```python
from build123d import *

# Parameters (mm, degrees)
ESQUISSE1_R                  = 100
BOSS_EXTRU_1_DEPTH           = 10
ENL_V_MAT_EXTRU_1_DEPTH      = 142.774468788
ENL_V_MAT_EXTRU_1_DEPTH_BACK = 142.774468788
CONG_1_R                     = 5
ENL_V_MAT_EXTRU_2_DEPTH      = 142.774468788
ENL_V_MAT_EXTRU_2_DEPTH_BACK = 142.774468788
ESQUISSE3_R                  = 8
ENL_V_MAT_EXTRU_3_DEPTH      = 142.774468788
ENL_V_MAT_EXTRU_3_DEPTH_BACK = 142.774468788
ESQUISSE4_R                  = 2.1
ENL_V_START                  = 100
ESQUISSE5_R                  = 3
ENL_V_MAT_EXTRU_4_DEPTH      = 10
R_P_TITION_CIRCULAIRE1_COUNT = 6


with BuildPart() as part:
    # Esquisse1 → Boss.-Extru.1 (new body)
    with BuildSketch(Plane.XY):
        Circle(ESQUISSE1_R)
    extrude(amount=BOSS_EXTRU_1_DEPTH)

    # Esquisse2 → Enlèv. mat.-Extru.1 (cut, two sides: drawn at the far end of the back side and taken through both)
    with BuildSketch(Plane.XY.offset(10).offset(-ENL_V_MAT_EXTRU_1_DEPTH_BACK)):
        with BuildLine():
            Line((10, 0), (80.321912081, 40.60037487))
            ThreePointArc((80.321912081, 40.60037487), (90, 0), (80.321912081, -40.60037487))
            Line((80.321912081, -40.60037487), (10, 0))
        make_face()
        with BuildLine():
            Line((5, -8.660254038), (75.321912081, -49.260628908))
            ThreePointArc((75.321912081, -49.260628908), (45, -77.942286341), (5, -89.861003778))
            Line((5, -89.861003778), (5, -8.660254038))
        make_face()
        with BuildLine():
            Line((-5, -8.660254038), (-5, -89.861003778))
            ThreePointArc((-5, -89.861003778), (-45, -77.942286341), (-75.321912081, -49.260628908))
            Line((-75.321912081, -49.260628908), (-5, -8.660254038))
        make_face()
        with BuildLine():
            Line((-10, 0), (-80.321912081, -40.60037487))
            ThreePointArc((-80.321912081, -40.60037487), (-90, 0), (-80.321912081, 40.60037487))
            Line((-80.321912081, 40.60037487), (-10, 0))
        make_face()
        with BuildLine():
            Line((-5, 8.660254038), (-75.321912081, 49.260628908))
            ThreePointArc((-75.321912081, 49.260628908), (-45, 77.942286341), (-5, 89.861003778))
            Line((-5, 89.861003778), (-5, 8.660254038))
        make_face()
        with BuildLine():
            Line((5, 8.660254038), (5, 89.861003778))
            ThreePointArc((5, 89.861003778), (45, 77.942286341), (75.321912081, 49.260628908))
            Line((75.321912081, 49.260628908), (5, 8.660254038))
        make_face()
    extrude(amount=ENL_V_MAT_EXTRU_1_DEPTH + ENL_V_MAT_EXTRU_1_DEPTH_BACK, mode=Mode.SUBTRACT)

    # Congé1
    cong_1_edges = [part.edges().sort_by_distance(p)[0] for p in [
        (80.321912081, -40.60037487, 5),
        (10, 0, 5),
        (80.321912081, 40.60037487, 5),
        (-80.321912081, 40.60037487, 5),
        (-10, 0, 5),
        (-80.321912081, -40.60037487, 5),
        (-5, 89.861003778, 5),
        (-5, 8.660254038, 5),
        (-75.321912081, 49.260628908, 5),
        (75.321912081, 49.260628908, 5),
        (5, 8.660254038, 5),
        (5, 89.861003778, 5),
        (-75.321912081, -49.260628908, 5),
        (-5, -8.660254038, 5),
        (-5, -89.861003778, 5),
        (5, -89.861003778, 5),
        (5, -8.660254038, 5),
        (75.321912081, -49.260628908, 5),
    ]]
    fillet(cong_1_edges, radius=CONG_1_R)

    # Esquisse3 → Enlèv. mat.-Extru.2 (cut, two sides: drawn at the far end of the back side and taken through both)
    with BuildSketch(Plane.XY.offset(10).offset(-ENL_V_MAT_EXTRU_2_DEPTH_BACK)):
        Circle(ESQUISSE3_R)
    extrude(amount=ENL_V_MAT_EXTRU_2_DEPTH + ENL_V_MAT_EXTRU_2_DEPTH_BACK, mode=Mode.SUBTRACT)

    # Esquisse4 → Enlèv. mat.-Extru.3 (cut, two sides: drawn at the far end of the back side and taken through both)
    with BuildSketch(Plane.XY.offset(10).offset(-ENL_V_MAT_EXTRU_3_DEPTH_BACK)):
        with Locations((0, 12)):
            Circle(ESQUISSE4_R)
        with Locations((10.392304845, -6)):
            Circle(ESQUISSE4_R)
        with Locations((-10.392304845, -6)):
            Circle(ESQUISSE4_R)
    extrude(amount=ENL_V_MAT_EXTRU_3_DEPTH + ENL_V_MAT_EXTRU_3_DEPTH_BACK, mode=Mode.SUBTRACT)

    # Esquisse5 → Enlèv. mat.-Extru.4 (cut)
    with BuildSketch(Plane(origin=(0, 0, 0), x_dir=(0, 0, -1), z_dir=(0, 1, 0)).offset(ENL_V_START)):
        with Locations(Location((-5, 0, 0), (0, 0, 180))):
            Circle(ESQUISSE5_R)
    enl_v_mat_extru_4 = extrude(amount=-ENL_V_MAT_EXTRU_4_DEPTH, mode=Mode.SUBTRACT)

    # Répétition circulaire1: Enlèv. mat.-Extru.4 ×6 about axis
    r_p_tition_circulaire1_axis = Axis((0, 0, 0), (0, 0, 1))
    for i in range(1, R_P_TITION_CIRCULAIRE1_COUNT):
        add(enl_v_mat_extru_4.rotate(r_p_tition_circulaire1_axis, i * 360 / R_P_TITION_CIRCULAIRE1_COUNT), mode=Mode.SUBTRACT)


solid = part.part
```
Source: CAD feature listing. Evaluate the final solid. Frame: model axes, mm. A direction names the side the tool comes from. Round coordinates to 2 decimals unless told otherwise and drop trailing zeros. Loops run counter-clockwise (first coordinate to the right, second up) from the corner with the lowest first, then second, coordinate; pieces in that order, holes last.
(1) Access query for faces 1 (the flat face through (-77.92, 45.04, 4.96)), 2 (the flat face through (-46.96, 21.34, 4.93)). Directions: +Z, -Z, +X, -X, +Y, -Y. A direction counts if a zero-diameter tool reaches every point of the face in a straight line with its end or side. Return the directions, or none.
From the geometry:
face 1: none
face 2: +Z, -Z
(2) Material intervals for probe 1 along Y at (x, z) = (51.5, 1.25); probe 2 along Y at (x, z) = (0, 6.75); probe 3 along X at (y, z) = (-77, 6.75), sorted ascending.
From the geometry:
probe 1: y = -85.72 to -73.81, -35.51 to -23.96, 23.96 to 35.51, 73.81 to 85.72
probe 2: y = -90 to -8, 8 to 9.9, 14.1 to 90
probe 3: x = -63.8 to -46.59, -5 to 5, 46.59 to 63.8
(3) Section query B-B (x = -63). Output: boundary loops of the cut face in (y, z), and give its area (3 significant figures).
From the geometry:
outline: (-77.66, 0) - (-64.27, 0) - (-64.27, 10) - (-77.66, 10) - close; (-42.15, 0) - (-30.6, 0) - (-30.6, 10) - (-42.15, 10) - close; (30.6, 0) - (42.15, 0) - (42.15, 10) - (30.6, 10) - close; (64.27, 0) - (77.66, 0) - (77.66, 10) - (64.27, 10) - close
area: 499 mm2
(4) Section query C-C (y = -76.5). Output: boundary loops of the cut face in (x, z).
From the geometry:
outline: (-64.4, 0) - (-47.41, 0) - (-47.41, 10) - (-64.4, 10) - close; (-5, 0) - (5, 0) - (5, 10) - (-5, 10) - close; (47.41, 0) - (64.4, 0) - (64.4, 10) - (47.41, 10) - close
(5) Section query D-D (z = 6.25). Give the number of separate pieces and of enclosed holes in the cut face, and give its area (3 significant figures).
From the geometry:
separate pieces: 1
enclosed holes: 10
area: 10,700 mm2
(6) Section query A-A (y = 71). Output: boundary loops of the cut face in (x, z), and give its area (3 significant figures).
From the geometry:
outline: (-70.42, 0) - (-55.31, 0) - (-55.31, 10) - (-70.42, 10) - close; (-5, 0) - (5, 0) - (5, 10) - (-5, 10) - close; (55.31, 0) - (70.42, 0) - (70.42, 10) - (55.31, 10) - close
area: 402 mm2
(7) Contact query for flat-ended pins moving along their axis: pin 1 Ø3.5 at (x, z) = (0, 5) entering from -Y; pin 2 Ø2 at (y, z) = (-27, 6) entering from -X; pin 3 Ø3 at (x, z) = (59.5, 6) entering from +Y. Output: stop coordinate, or through.
From the geometry:
pin 1: stops at y = -90
pin 2: stops at x = -96.56
pin 3: stops at y = 81.46
